The drawing under review shows one solid part. Ordinate dimensions are in mm from its lowest x, y, z. Round coordinates to 2 decimals unless told otherwise and drop trailing zeros. Write each loop counter-clockwise with the first axis right and the second up, starting at its lowest first coordinate (ties: lowest second). Pieces come first, ordered by that corner, then holes. Notation, with made-up numbers: M -24.75,32.25 L -0.75,32.25 A35 cw -0.75,65.25 Z; hole C 61.5,68.25 d8. An arc over 180 degrees is marked long. Write item = value, one per line. Start each with the question number.
Item 1: Take a section at A-A, the plane x = 19.65. Give the boundary of the cut face in (y, z), plus the area to 3 significant figures.
Item 2: To check wall thickness, follow line 1 along Y through (x, z) = (19.65, 1.5); line 2 along Y through (x, z) = (50, 2.45); line 3 along X through (y, z) = (27.5, 0.4). State the ranges of each line that lie inside material, in increasing order.
Item 3: For pin 1 Ø7 at (x, y) = (19.65, 22.1) entering from +Z; pin 2 Ø0.9 at (x, z) = (48, 2) entering from +Y; pin 3 Ø0.9 at (y, z) = (2.5, 2) entering from -X, all flat-tipped, find the tip position at first contact; note any pin that passes through.
Item 4: Take a section at B-B, the plane y = 22.1. Give the boundary of the cut face in (x, z).
Item 5: Take a section at D-D, the plane x = 8.5. Give the boundary of the cut face in (y, z).
Item 6: Take a section at C-C, the plane z = 2.5. Give the boundary of the cut face in (x, y), plus the area to 3 significant figures.
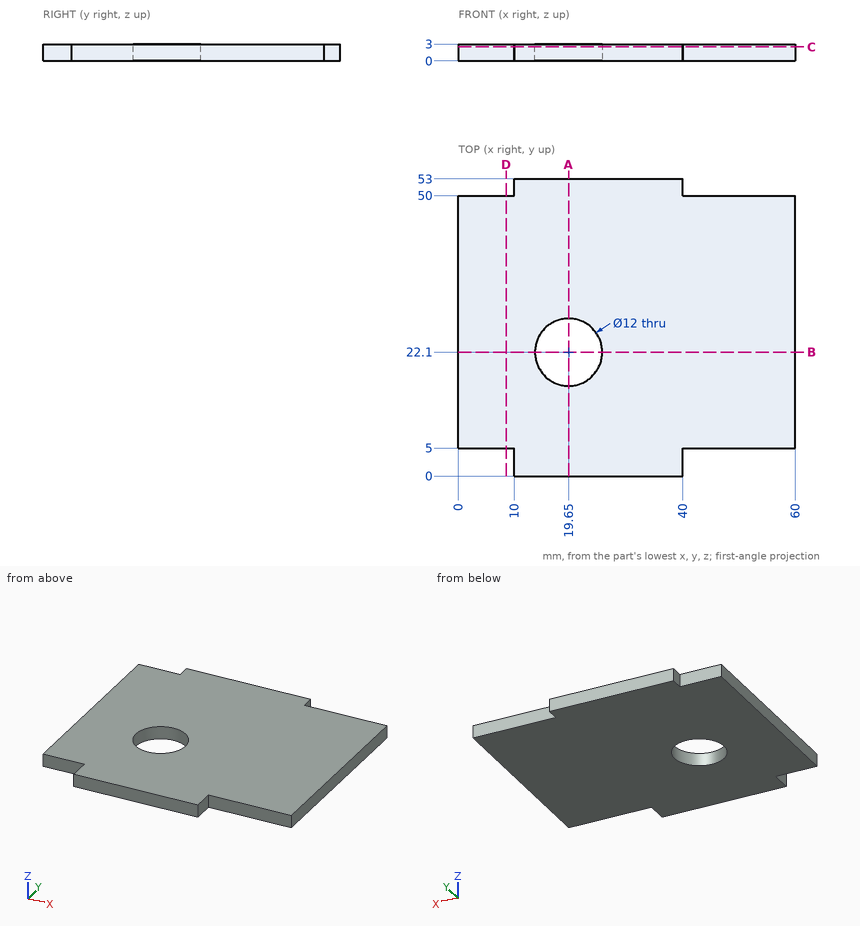
Response values:
q1.outline = M 0,0 L 16.1,0 L 16.1,3 L 0,3 Z; M 28.1,0 L 53,0 L 53,3 L 28.1,3 Z
q1.area = 123 mm2
q2.line_1 = 0 to 16.1, 28.1 to 53
q2.line_2 = 5 to 50
q2.line_3 = 0 to 17.03, 22.27 to 60
q3.pin_1 = through
q3.pin_2 = 50
q3.pin_3 = 10
q4.outline = M 0,0 L 13.65,0 L 13.65,3 L 0,3 Z; M 25.65,0 L 60,0 L 60,3 L 25.65,3 Z
q5.outline = M 5,0 L 50,0 L 50,3 L 5,3 Z
q6.outline = M 0,5 L 10,5 L 10,0 L 40,0 L 40,5 L 60,5 L 60,50 L 40,50 L 40,53 L 10,53 L 10,50 L 0,50 Z; hole C 19.65,22.1 d12
q6.area = 2,830 mm2
